from build123d import *

# Parameters (mm, degrees)
SKETCH_3_W    = 45
SKETCH_3_H    = 12
BAR_DEPTH     = 16
SKETCH_4_R    = 11
ROOTHUB_DEPTH = 26
SKETCH_5_R    = 10
ENDHUB_DEPTH  = 18


with BuildPart() as part:
    # 草图3 → Bar (new body)
    with BuildSketch(Plane.XY):
        with Locations((42.5, 12)):
            Rectangle(SKETCH_3_W, SKETCH_3_H)
    extrude(amount=BAR_DEPTH)

    # 草图4 → RootHub (add)
    with BuildSketch(Plane.XY):
        with Locations(Location((20, 12, 0), (0, 0, 326.944268849))):
            Circle(SKETCH_4_R)
    extrude(amount=ROOTHUB_DEPTH)

    # 草图5 → EndHub (add)
    with BuildSketch(Plane.XY):
        with Locations(Location((65, 12, 0), (0, 0, 216.869897646))):
            Circle(SKETCH_5_R)
    extrude(amount=ENDHUB_DEPTH)


solid = part.part
Source: CAD feature listing. Evaluate the final solid. Frame: model axes, mm. A direction names the side the tool comes from. Give positions to 0.01 mm unless a question says otherwise; leave off trailing zeros. Write each loop counter-clockwise with the first axis right and the second up, starting at its lowest first coordinate (ties: lowest second). Pieces come first, ordered by that corner, then holes. Notation, with made-up numbers: (47, -31) - (52, -31) arc R21 cw to (52, -25) - close; hole circle Ø5 at (55.5, 75). An arc over 180 degrees is marked (long way). Write item = value, one per line. Start each with the question number.
Q1. Cut plane B-B, the plane z = 11.25. Return loops of the section in (x, y).
Q2. Cut plane C-C, the plane x = 51. Return loops of the section in (y, z).
Q3. Cut plane D-D, the plane z = 23.5. Return loops of the section in (x, y).
Q4. Cut plane A-A, the plane y = 12. Return loops of the section in (x, z).
Q5. Draft query along X for faces 4 (the cylindrical face through (9.033, 11.151, 12.818)), 5 (the flat face through (43, 12, 16)), 6 (the flat face through (65, 12, 18)). Return one class per face: +X half, -X half, draft (parallel to the pull), parting line (faces both ways), or undercut.
Q6. Material intervals for probe 1 along Y at (x, z) = (30.5, 14.25); probe 2 along Z at (x, y) = (31, 16.75); probe 3 along X at (y, z) = (3.25, 17), sorted ascending.
Q7. Pin query (flat end, axial travel): pin 1 Ø5 at (y, z) = (18.5, 5.5) entering from +X; pin 2 Ø6 at (x, y) = (40, 12.5) entering from +Z; pin 3 Ø10 at (y, z) = (17.5, 23.5) entering from -X. Return the tip coordinate at first contact, or that it passes through.
Q8. Reachability of faces 1 (the flat face through (43, 6, 8)), 2 (the flat face through (42, 12, 0)), 3 (the flat face through (43, 18, 8)) from +Z, -Z, +X, -X, +Y, -Y: full face, straight path, thin tool, end or side. Return the list, or none.
Computed values:
q1.outline = (29.22, 6) - (57, 6) arc R10 ccw (long way) to (57, 18) - (29.22, 18) arc R11 ccw (long way) to start
q2.outline = (6, 0) - (18, 0) - (18, 16) - (6, 16) - close
q3.outline = circle Ø22 at (20, 12)
q4.outline = (9, 0) - (75, 0) - (75, 18) - (55, 18) - (55, 16) - (31, 16) - (31, 26) - (9, 26) - close
q5.face_4 = undercut
q5.face_5 = undercut
q5.face_6 = draft
q6.probe_1 = 6 to 18
q6.probe_2 = 0 to 16
q6.probe_3 = 13.33 to 26.67, 60.16 to 69.84
q7.pin_1 = 74.17
q7.pin_2 = 16
q7.pin_3 = 9.01
q8.face_1 = +Z, -Z, -Y
q8.face_2 = -Z, +X, -X, +Y, -Y
q8.face_3 = +Z, -Z, +Y
